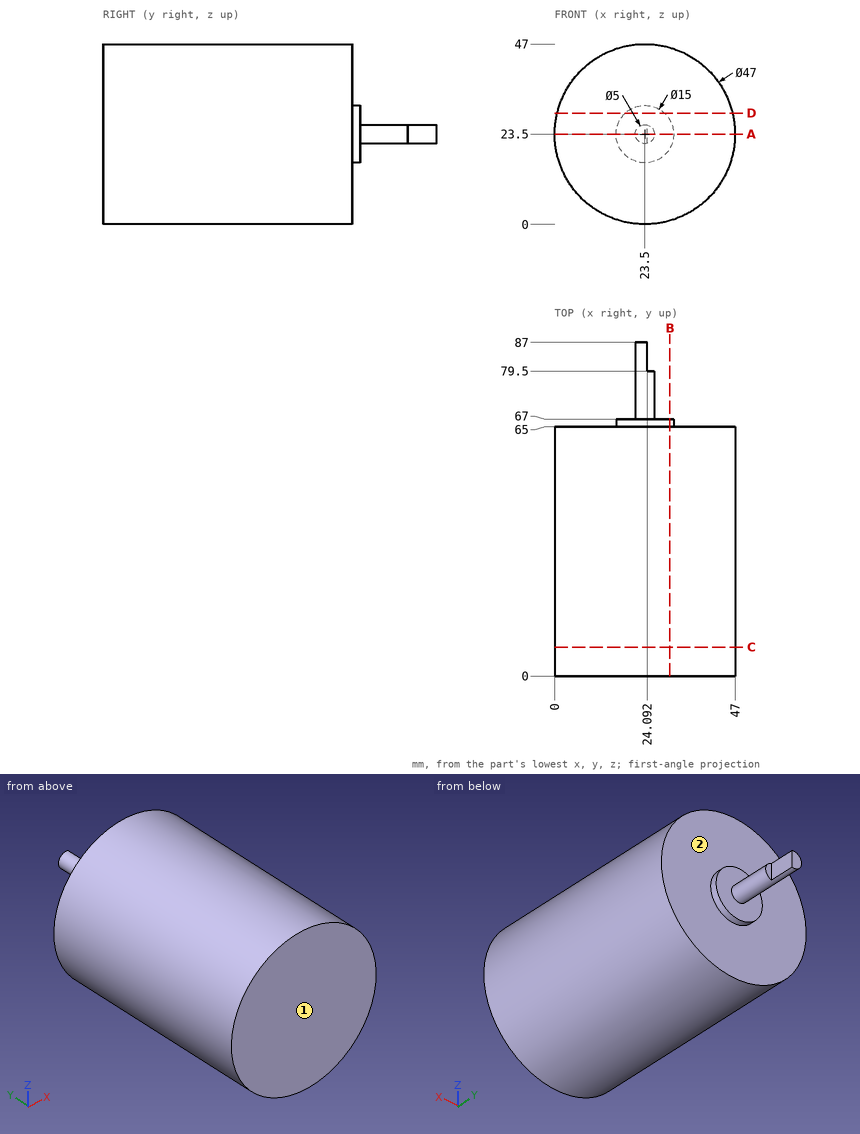
Source: three-view drawing plus pictorial views. Frame: mm from the lowest corner of the part. A direction names the side the tool comes from. Coordinates: 2 decimals unless noted, no trailing zeros. Order: outer loops, then holes, each group sorted by start corner. A loop starts at its lowest first (then second) coordinate and runs counter-clockwise, first axis right, second up.
Item 1: Cut plane B-B (x = 30). Return loops of the section in (y, z).
Output values:
outline: (0, 0.92) - (65, 0.92) - (65, 19.76) - (67, 19.76) - (67, 27.24) - (65, 27.24) - (65, 46.08) - (0, 46.08) - close
Item 2: Cut plane D-D (z = 29). Return loops of the section in (x, y).
Output values:
outline: (0.65, 0) - (46.35, 0) - (46.35, 65) - (28.6, 65) - (28.6, 67) - (18.4, 67) - (18.4, 65) - (0.65, 65) - close
Item 3: Cut plane C-C (y = 7.5). Return loops of the section in (x, z).
Output values:
outline: circle Ø47 at (23.5, 23.5)
Item 4: Material intervals for line 1 (Y direction, x = 18, z = 18.5); line 2 (Y direction, x = 31.5, z = 2.5); line 3 (Z direction, x = 4, y = 20.5) (3 decimals), sorted ascending.
Output values:
line 1: y = 0 to 67
line 2: y = 0 to 65
line 3: z = 10.385 to 36.615
Item 5: Set-up query: the marked faces 1 and 2. Return all of +Z, -Z, +X, -X, +Y, -Y with unobstructed straight access to the full face (end or side cutting, diameter ignored); none if empty.
Output values:
face 1: +Z, -Z, +X, -X, -Y
face 2: +Y
Item 6: First-contact query: P1, Ø6, axis at x = 12, y = 33, coming from the +Z side; P2, Ø1.5, axis at x = 11.5, y = 33, coming from the +Z side; P3, Ø10, axis at x = 18, y = 31, coming from the -Z side; P4, Ø12, axis at x = 25, z = 23.5, coming from the +Y side. Flat tips, straight axial feed; report the tip coordinate or a pass-through.
Output values:
P1: stops at z = 45.41
P2: stops at z = 44.13
P3: stops at z = 0.01
P4: stops at y = 87
Item 7: Cut plane A-A (z = 23.5). Return loops of the section in (x, y), plus the area to 3 significant figures.
Output values:
outline: (0, 0) - (47, 0) - (47, 65) - (31, 65) - (31, 67) - (26, 67) - (26, 79.5) - (24.09, 79.5) - (24.09, 87) - (21, 87) - (21, 67) - (16, 67) - (16, 65) - (0, 65) - close
area: 3,170 mm2
